Here's how the part is built. I have some questions about the finished solid (model axes, mm). A direction names the side the tool comes from. Round coordinates to 2 decimals unless told otherwise and drop trailing zeros. Order: outer loops, then holes, each group sorted by start corner. A loop starts at its lowest first (then second) coordinate and runs counter-clockwise, first axis right, second up.
```python
from build123d import *

# Parameters (mm, degrees)
EXTRUDE_1_DEPTH     = 3
EXTRUDE_2_DEPTH     = 3
SKETCH_3_R          = 2.5
CUT_EXTRUDE_1_DEPTH = 3
EXTRUDE_3_DEPTH     = 3
SKETCH_5_R          = 2.5
CUT_EXTRUDE_2_DEPTH = 108.032497136


with BuildPart() as part:
    # Sketch 1 → Extrude 1 (new body)
    with BuildSketch(Plane.XY):
        with BuildLine():
            ThreePointArc((2.49494029, -11.737771209), (38.552147634, 2.82859918), (67.45494029, 28.846476198))
            ThreePointArc((67.45494029, 28.846476198), (65.389458987, 45.690875474), (48.54505971, 43.625394171))
            ThreePointArc((48.54505971, 43.625394171), (25.835722623, 23.182776515), (-2.49494029, 11.737771209))
            ThreePointArc((-2.49494029, 11.737771209), (-11.737771209, -2.49494029), (2.49494029, -11.737771209))
        make_face()
        with BuildLine():
            ThreePointArc((1.039558454, -4.890738004), (34.843190339, 8.765234236), (61.939558454, 33.15699394))
            ThreePointArc((61.939558454, 33.15699394), (61.078941244, 40.175493638), (54.060441546, 39.314876429))
            ThreePointArc((54.060441546, 39.314876429), (29.544679918, 17.246141459), (-1.039558454, 4.890738004))
            ThreePointArc((-1.039558454, 4.890738004), (-4.890738004, -1.039558454), (1.039558454, -4.890738004))
        make_face(mode=Mode.SUBTRACT)
    extrude(amount=EXTRUDE_1_DEPTH)

    # Sketch 2 → Extrude 2 (add)
    with BuildSketch(Plane.XY):
        with BuildLine():
            ThreePointArc((89.676000633, 32.310336646), (77.132851548, 37.028551056), (66.293420251, 44.908834385))
            ThreePointArc((66.293420251, 44.908834385), (69.968747349, 37.101433246), (67.45494029, 28.846476198))
            ThreePointArc((67.45494029, 28.846476198), (57.764135997, 17.983287307), (46.746204448, 8.468785476))
            ThreePointArc((46.746204448, 8.468785476), (65.669563572, 17.30537468), (86.551758878, 17.641155141))
            ThreePointArc((86.551758878, 17.641155141), (95.33547477, 23.437690844), (89.676000633, 32.310336646))
        make_face()
    extrude(amount=EXTRUDE_2_DEPTH)

    # Sketch 3 → Cut-Extrude 1 (cut)
    with BuildSketch(Plane.XY.offset(3)):
        with Locations((88, 25)):
            Circle(SKETCH_3_R)
    extrude(amount=-CUT_EXTRUDE_1_DEPTH, mode=Mode.SUBTRACT)

    # Sketch 4 → Extrude 3 (add)
    with BuildSketch(Plane.XY):
        with BuildLine():
            ThreePointArc((86.551758798, 17.641155157), (73.513996149, 18.467623485), (60.707166945, 15.888586743))
            ThreePointArc((60.707166945, 15.888586743), (74.740298782, 13.562445033), (80.52135397, 0.56555597))
            ThreePointArc((80.52135397, 0.56555597), (80.505340394, 0.282979481), (80.5, 0))
            ThreePointArc((80.5, 0), (89.268264866, -7.391989193), (95.071067795, 2.500000049))
            ThreePointArc((95.071067795, 2.500000049), (93.355339059, 12.500000074), (95.071067844, 22.500000091))
            ThreePointArc((95.071067844, 22.500000091), (91.715661231, 18.485104635), (86.551758798, 17.641155157))
        make_face()
    extrude(amount=EXTRUDE_3_DEPTH)

    # Sketch 5 → Cut-Extrude 2 (cut, through all)
    with BuildSketch(Plane.XY.offset(3)):
        with Locations((88, 0)):
            Circle(SKETCH_5_R)
    extrude(amount=-CUT_EXTRUDE_2_DEPTH, mode=Mode.SUBTRACT)


solid = part.part
```
1) For faces 4 (the cylindrical face through (25.418, -4.208, 1.479)), 5 (the cylindrical face through (57.275, 48.214, 1.479)), 6 (the cylindrical face through (34.407, 8.494, 1.479)), which set-ups out of +Z, -Z, +X, -X, +Y, -Y let a thin tool reach every point of the face, with its end or its side?
2) I need wall thicknesses on line 1 (X direction, y = 4, z = 2.25); line 2 (Y direction, x = 88, z = 2.2); line 3 (Y direction, x = 14, z = 0.8). Which ranges of each line are inside material? Lowest first, please.
3) If we section it at A-A (z = 2.4): Write out the boundary of the cut face in (x, y).
4) If we section it at C-C (y = 25): Write out the boundary of the cut face in (x, z).
5) If we section it at D-D (x = 88): Write out the boundary of the cut face in (y, z).
6) If we section it at B-B (x = 27): Write out the boundary of the cut face in (y, z).
7) We'd pull the mould along Y, two halves only. Please class faces 1 (the flat face through (53, 19, 3)), 2 (the cylindrical face through (77.3, 36.94, 1.48)), 3 (the cylindrical face through (29.938, 17.493, 1.479)): +Y half, -Y half, draft (parallel to the pull), parting line (faces both ways), or undercut.
Solutions:
1. face 4: +Z, -Z, -Y
1. face 5: +Z, -Z, +Y
1. face 6: +Z, -Z
2. line 1: x = -11.31 to -3, 26.37 to 40.39, 80.39 to 94.58
2. line 2: y = -7.5 to -2.5, 2.5 to 22.5, 27.5 to 32.73
2. line 3: y = -8.64 to -1.25, 9.41 to 16.98
3. outline: (-2.49, 11.74) arc R12 ccw to (2.49, -11.74) arc R112 ccw to (46.75, 8.47) arc R50 cw to (60.71, 15.89) arc R15 cw to (80.52, 0.57) arc R7.5 ccw (long way) to (95.07, 2.5) arc R30 cw to (95.07, 22.5) arc R7.5 ccw to (89.68, 32.31) arc R50 cw to (66.29, 44.91) arc R12 ccw to (48.55, 43.63) arc R88 cw to start; hole (-1.04, 4.89) arc R5 ccw to (1.04, -4.89) arc R105 ccw to (61.94, 33.16) arc R5 ccw to (54.06, 39.31) arc R95 cw to start; hole circle Ø5 at (88, 0); hole circle Ø5 at (88, 25)
4. outline: (28.63, 0) - (40.23, 0) - (40.23, 3) - (28.63, 3) - close; (54.86, 0) - (85.5, 0) - (85.5, 3) - (54.86, 3) - close; (90.5, 0) - (95.5, 0) - (95.5, 3) - (90.5, 3) - close
5. outline: (-7.5, 0) - (-2.5, 0) - (-2.5, 3) - (-7.5, 3) - close; (2.5, 0) - (22.5, 0) - (22.5, 3) - (2.5, 3) - close; (27.5, 0) - (32.73, 0) - (32.73, 3) - (27.5, 3) - close
6. outline: (-3.48, 0) - (4.32, 0) - (4.32, 3) - (-3.48, 3) - close; (15.71, 0) - (23.92, 0) - (23.92, 3) - (15.71, 3) - close
7. face 1: draft
7. face 2: +Y half
7. face 3: undercut
